The drawing under review shows one solid part. Ordinate dimensions are in mm from its lowest x, y, z. Give positions to 0.01 mm unless a question says otherwise; leave off trailing zeros. Order: outer loops, then holes, each group sorted by start corner. A loop starts at its lowest first (then second) coordinate and runs counter-clockwise, first axis right, second up. Notation, with made-up numbers: (24.25, -37.5) - (61.25, -37.5) arc R24 ccw to (61.25, -22.5) - close; hole circle Ø3 at (28, 85.25). An arc over 180 degrees is marked (long way). Use CSV: the item, a comma, the result in double quotes. Start each with the question number.
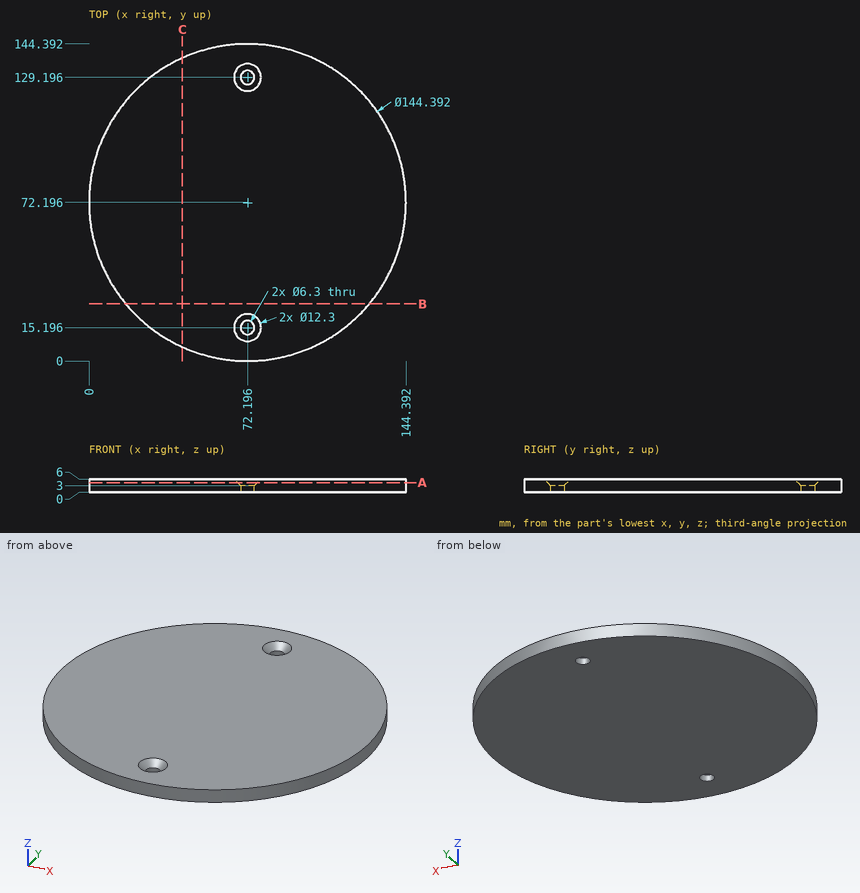
1. Consider section C-C (x = 42.5). Give the boundary of the cut face in (y, z).
2. To check wall thickness, follow L1, parallel to Y at x = 72, z = 0.7; L2, parallel to Y at x = 70.5, z = 5.75 (1 decimal); L3, parallel to X at y = 18, z = 2.25 (1 decimal). State the ranges of each line that lie inside material, in increasing order. Write a range as [from, to].
3. Consider section A-A (z = 4.35). Give the boundary of the cut face in (x, y) (1 decimal), and give its area (3 significant figures).
4. Clearance check with flat-ended pins moving along their axes: pin 1 (1 mm diameter, centred on x = 27.5, z = 5, fed in from +Y); pin 2 (1.5 mm diameter, centred on y = 53, z = 1, fed in from +X) (1 decimal); pin 3 (2 mm diameter, centred on y = 118, z = 4, fed in from -X) (1 decimal); pin 4 (5 mm diameter, centred on x = 72.2, y = 129.2, fed in from +Z). State where each tip first meets the part, or that it passes through.
5. Consider section B-B (y = 26). Give the boundary of the cut face in (x, z) (1 decimal), and give its area (3 significant figures).
Answers follow:
1,outline,"(6.39, 0) - (138, 0) - (138, 6) - (6.39, 6) - close"
2,L1,"y = [0, 12.05], [18.34, 126.05], [132.34, 144.39]"
2,L2,"y = [0, 9.5], [20.8, 123.5], [134.8, 144.4]"
2,L3,"x = [24.5, 70.8], [73.6, 119.9]"
3,outline,"circle Ø144.4 at (72.2, 72.2); hole circle Ø9 at (72.2, 15.2); hole circle Ø9 at (72.2, 129.2)"
3,area,"16,200 mm^2"
4,pin 1,"stops at y = 129.28"
4,pin 2,"stops at x = 142"
4,pin 3,"stops at x = 15.6"
4,pin 4,"passes through"
5,outline,"(16.7, 0) - (127.7, 0) - (127.7, 6) - (16.7, 6) - close"
5,area,"666 mm^2"
